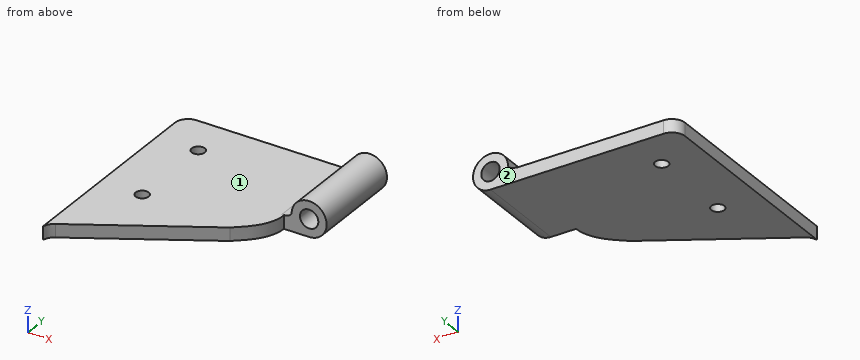
from build123d import *

# Parameters (mm, degrees)
F1_DEPTH = 3
F2_R     = 2.1
F3_DEPTH = 21.5
F4_R     = 3
F5_R     = 1.5
F6_DEPTH = 3


with BuildPart() as f1:
    # F0 (on Top) → F1 (new body)
    with BuildSketch(Plane.XY):
        with BuildLine():
            add(Edge.make_bspline(
                [(-17.7381685377, 25.758469689), (-18.6029082943, 25.3198112197), (-19.0115179867, 24.4438797075), (-19.25, 23.7522523094)],
                knots=[0, 0, 0, 0, 2.5120793269, 2.5120793269, 2.5120793269, 2.5120793269], degree=3))
            Line((-17.7381685377, 25.758469689), (11.2471123299, 42.7481702213))
            add(Edge.make_bspline(
                [(11.2471123299, 42.7481702213), (13.6908411554, 44.7339186325), (17.38480106, 47.4555082619), (17.5, 52.2522523094)],
                knots=[0, 0, 0, 0, 11.376562774, 11.376562774, 11.376562774, 11.376562774], degree=3))
            Line((17.5, 52.2522523094), (19.25, 52.2522523094))
            Line((19.25, 52.2522523094), (19.25, 73.7522523094))
            Line((19.25, 73.7522523094), (-19.25, 73.7522523094))
            Line((-19.25, 73.7522523094), (-19.25, 23.7522523094))
        make_face()
    extrude(amount=F1_DEPTH)

    # F2 (on face) → F3 (join)
    with BuildSketch(Plane(origin=(0, 73.7522523094, 0), x_dir=(-1, 0, 0), z_dir=(0, 1, 0))):
        with BuildLine():
            ThreePointArc((-23.25, 0), (-20.4215728753, 1.1715728753), (-19.25, 4))
            ThreePointArc((-19.25, 4), (-26.0784271247, 6.8284271247), (-23.25, 0))
        make_face()
        with Locations((-23.25, 4)):
            Circle(F2_R, mode=Mode.SUBTRACT)
        with BuildLine():
            Line((-23.25, 0), (-19.25, 0))
            Line((-19.25, 0), (-19.25, 3))
            Line((-19.25, 3), (-16.9664081186, 3))
            add(Edge.make_bspline(
                [(-19.25, 4), (-18.8806392252, 3.1797552947), (-18.1370340288, 3.1503054779), (-16.9664081186, 3)],
                knots=[0, 0, 0, 0, 2.4929484312, 2.4929484312, 2.4929484312, 2.4929484312], degree=3))
            ThreePointArc((-19.25, 4), (-20.4215728753, 1.1715728753), (-23.25, 0))
        make_face()
    extrude(amount=-F3_DEPTH)

    # F4
    f4_edges = [f1.edges().sort_by_distance(p)[0] for p in [
        (-19.25, 73.752252, 1.5),
    ]]
    fillet(f4_edges, radius=F4_R)

    # F5 (on face) → F6 (cut)
    with BuildSketch(Plane(origin=(0, 0, 0), x_dir=(1, 0, 0), z_dir=(0, 0, -1))):
        with Locations((-9.75, -64.2522523094)):
            Circle(F5_R)
        with Locations((-9.75, -44.2522523094)):
            Circle(F5_R)
    extrude(amount=-F6_DEPTH, mode=Mode.SUBTRACT)


solid = f1.part
Verification items for the finished model (mm, model axes). Face numbers are marked on the shaded views. A direction names the side the tool comes from. Coordinates: 2 decimals unless noted, no trailing zeros. Order: outer loops, then holes, each group sorted by start corner. A loop starts at its lowest first (then second) coordinate and runs counter-clockwise, first axis right, second up. Notation, with made-up numbers: (47.5, 18.25) -> (73.5, 18.25) arc R8 cw to (73.5, 29.25) -> close; hole circle Ø10 at (48.25, 14). An arc over 180 degrees is marked (long way). Use CSV: the item, a comma, the result in double quotes. Start each with the question number.
Q1. Section check C-C, the plane x = 1.5. Record the cut outline in (y, z).
Q2. Tool access check on the marked faces 1 and 2. Record the directions out of +Z, -Z, +X, -X, +Y, -Y that give a thin tool (end or side, any length) a straight path to the whole face; none if there is none.
Q3. Section check B-B, the plane z = 1.25. Give the number of separate pieces and of enclosed holes in the cut face, and give its area (3 significant figures).
Q4. Thickness scan on line 1 along Y through (x, z) = (-10.5, 1); line 2 along Y through (x, z) = (-9.75, 1.95); line 3 along Z through (x, y) = (15.5, 67.5). Record the ranges inside material, lowest first.
Q5. Depth check by flat-ended pin: P1, Ø4, axis at x = -9.75, y = 44.25, coming from the +Z side; P2, Ø5, axis at x = -5, y = 48.5, coming from the -Z side; P3, Ø4, axis at x = 24, z = 5.5, coming from the -Y side. Enter the tip coordinate at first touch or a pass-through.
Q6. Section check D-D, the plane y = 34.5. Record the cut outline in (x, z).
Q7. Section check A-A, the plane x = -9.75. Record the cut outline in (y, z).
Returned:
1,outline,"(37.03, 0) -> (73.75, 0) -> (73.75, 3) -> (37.03, 3) -> close"
2,face 1,"+Z, -X, +Y, -Y"
2,face 2,"+Z, -Z, +X, -X, +Y"
3,separate pieces,"1"
3,enclosed holes,"2"
3,area,"1,560 mm^2"
4,line 1,"y = 30 to 42.95, 45.55 to 62.95, 65.55 to 73.75"
4,line 2,"y = 30.44 to 42.75, 45.75 to 62.75, 65.75 to 73.75"
4,line 3,"z = 0 to 3"
5,P1,"stops at z = 3"
5,P2,"stops at z = 0"
5,P3,"stops at y = 52.25"
6,outline,"(-19.25, 0) -> (-2.82, 0) -> (-2.82, 3) -> (-19.25, 3) -> close"
7,outline,"(30.44, 0) -> (42.75, 0) -> (42.75, 3) -> (30.44, 3) -> close; (45.75, 0) -> (62.75, 0) -> (62.75, 3) -> (45.75, 3) -> close; (65.75, 0) -> (73.75, 0) -> (73.75, 3) -> (65.75, 3) -> close"
